Read the model definition and answer for the solid it produces. Units are mm, in the model's axes. A direction names the side the tool comes from. Give positions to 0.01 mm unless a question says otherwise; leave off trailing zeros. Write each loop counter-clockwise with the first axis right and the second up, starting at its lowest first coordinate (ties: lowest second). Pieces come first, ordered by that corner, then holes.
```python
from build123d import *

# Parameters (mm, degrees)
F1_DEPTH = 70.975848
F3_DEPTH = 46.616317


with BuildPart() as f1:
    # F0 (on Top) → F1 (new body)
    with BuildSketch(Plane.XY):
        Polygon((0, 46.615317), (0, 0), (15, 0), (15, 34.846107), (45, 34.846107), (45, 0), (60, 0), (60, 46.615317), align=None)
    extrude(amount=F1_DEPTH)

    # F2 (on Front) → F3 (cut, through all)
    with BuildSketch(Plane.XZ):
        Polygon((60, 34.172569), (60, 70.975848), (30.000645, 71.172569), (30.000645, 34.172569), align=None)
    extrude(amount=-F3_DEPTH, mode=Mode.SUBTRACT)


solid = f1.part
```
Item 1: Which of the six approach directions +Z, -Z, +X, -X, +Y, -Y give full straight-line access (tool end or side, diameter ignored) to faces 1 (the flat face through (45, 18, 17)), 2 (the flat face through (30.001, 41, 53)), 3 (the flat face through (52, 0, 17))?
Result set:
face 1: +Z, -Z, -Y
face 2: +Z, +X, +Y, -Y
face 3: +Z, -Z, +X, -X, -Y
Item 2: Section C-C (x = 28.5) is taken. Write down the section's boundary in (y, z).
Result set:
outline: (34.85, 0) - (46.62, 0) - (46.62, 70.98) - (34.85, 70.98) - close
Item 3: Section A-A (y = 23) is taken. Write down the section's boundary in (x, z), and give its area (3 significant figures).
Result set:
outline: (0, 0) - (15, 0) - (15, 70.98) - (0, 70.98) - close; (45, 0) - (60, 0) - (60, 34.17) - (45, 34.17) - close
area: 1,580 mm2
Item 4: Determine the mould class of faces 4 (the flat face through (26, 34.846, 27)), 5 (the flat face through (0, 24, 35)), 6 (the flat face through (51, 28, 34.173)) for opening direction X: pulls with the +X half, pulls with the -X half, needs draft (parallel to the pull), parting line crosses it, or undercut.
Result set:
face 4: undercut
face 5: pulls with the -X half
face 6: needs draft
Item 5: Each of these flat-tipped pins is pushed along its axis until it touches: pin 1 Ø12 at (x, y) = (41, 16.5) entering from +Z; pin 2 Ø13 at (y, z) = (41, 45) entering from +X. Where does it stop, or does it pass through?
Result set:
pin 1: stops at z = 34.17
pin 2: stops at x = 30
Item 6: Find the intervals of material crossed by line 1 along X through (y, z) = (3, 23.5); line 2 along Y through (x, z) = (28.5, 63); line 3 along X through (y, z) = (12, 50.5), in increasing order.
Result set:
line 1: x = 0 to 15, 45 to 60
line 2: y = 34.85 to 46.62
line 3: x = 0 to 15
Item 7: Section D-D (y = 36) is taken. Write down the section's boundary in (x, z), and give its area (3 significant figures).
Result set:
outline: (0, 0) - (60, 0) - (60, 34.17) - (30, 34.17) - (30, 70.98) - (0, 70.98) - close
area: 3,150 mm2
Item 8: Section B-B (z = 31) is taken. Write down the section's boundary in (x, y).
Result set:
outline: (0, 0) - (15, 0) - (15, 34.85) - (45, 34.85) - (45, 0) - (60, 0) - (60, 46.62) - (0, 46.62) - close
